```python
from build123d import *

# Parameters (mm, degrees)
F0_R           = 4.75
F0_R_2         = 8.6
F1_DEPTH       = 15.5
F2_R           = 7.25
F3_DEPTH       = 8
F4_R           = 23.5
F4_R_2         = 8.6
F5_DEPTH       = 27
F6_R           = 15.875
F7_DEPTH       = 8
F8_R           = 15.875
F9_DEPTH       = 10
F14_R          = 3
F15_DEPTH      = 25
F15_DEPTH_BACK = 25
F16_R          = 3
F17_DEPTH      = 15.5


with BuildPart() as f1:
    # F0 (on Front) → F1 (new body)
    with BuildSketch(Plane.XZ):
        with BuildLine():
            ThreePointArc((-54.5, -13.8241850861), (-27.977340312, -23.2893113667), (0, -26.5))
            ThreePointArc((0, -26.5), (27.977340312, -23.2893113667), (54.5, -13.8241850861))
            Line((54.5, -13.8241850861), (54.5, 12.5))
            Line((54.5, 12.5), (47.5, 12.5))
            Line((47.5, 12.5), (47.5, 17))
            ThreePointArc((47.5, 17), (0, 26.5), (-47.5, 17))
            Line((-47.5, 17), (-47.5, 12.5))
            Line((-47.5, 12.5), (-54.5, 12.5))
            Line((-54.5, 12.5), (-54.5, -13.8241850861))
        make_face()
        with Locations((-40, 0)):
            Circle(F0_R, mode=Mode.SUBTRACT)
        Circle(F0_R_2, mode=Mode.SUBTRACT)
        with Locations((40, 0)):
            Circle(F0_R, mode=Mode.SUBTRACT)
    extrude(amount=F1_DEPTH)

    # F2 (on face) → F3 (cut)
    with BuildSketch(Plane.XZ.offset(15.5)):
        with Locations((-40, 0)):
            Circle(F2_R)
        with Locations((40, 0)):
            Circle(F2_R)
    extrude(amount=-F3_DEPTH, mode=Mode.SUBTRACT)

    # F4 (on face) → F5 (join)
    with BuildSketch(Plane.XZ.offset(15.5)):
        Circle(F4_R)
        Circle(F4_R_2, mode=Mode.SUBTRACT)
    extrude(amount=F5_DEPTH)

    # F6 (on face) → F7 (cut)
    with BuildSketch(Plane.XZ.offset(42.5)):
        Circle(F6_R)
    extrude(amount=-F7_DEPTH, mode=Mode.SUBTRACT)

    # F8 (on face) → F9 (cut)
    with BuildSketch(Plane(origin=(0, 0, 0), x_dir=(-1, 0, 0), z_dir=(0, 1, 0))):
        Circle(F8_R)
    extrude(amount=-F9_DEPTH, mode=Mode.SUBTRACT)

    # F14 (on 3pt) → F15 (cut, two sides)
    with BuildSketch(Plane.XY.offset(-0.6620925431)) as f15_sk:
        with Locations((0, -21.5)):
            Circle(F14_R)
    extrude(amount=F15_DEPTH, mode=Mode.SUBTRACT)
    extrude(f15_sk.sketch, amount=-F15_DEPTH_BACK, mode=Mode.SUBTRACT)

    # F16 (on face) → F17 (cut, through all)
    with BuildSketch(Plane.XZ.offset(15.5)):
        with Locations((-31.9875436575, 13.577906715)):
            Circle(F16_R)
        with Locations((31.9875436575, -13.577906715)):
            Circle(F16_R)
    extrude(amount=-F17_DEPTH, mode=Mode.SUBTRACT)


solid = f1.part
```
For this review, take the finished solid that the model builds, in its own axes (mm). A direction names the side the tool comes from. Give positions to 0.01 mm unless a question says otherwise; leave off trailing zeros. Loops run counter-clockwise (first coordinate to the right, second up) from the corner with the lowest first, then second, coordinate; pieces in that order, holes last. Notation, with made-up numbers: M -31,-6 L 10,-6 A15 ccw 10,11 Z; hole C -17.5,43 d4. An arc over 180 degrees is marked long. One line per item, written item: value. Start each with the question number.
Q1. Add section C-C (y = -21.5). Give the boundary of the cut face in (x, z).
Q2. Add section D-D (x = -18.5). Give the boundary of the cut face in (y, z).
Q3. Add section A-A (x = 40). Give the boundary of the cut face in (y, z).
Q4. Draft analysis for pull direction Z (two halves, no side actions). For faces 4 (the face through (44.53, -3.7, 1.43)), 5 (the face through (-0.65, -24.43, 15.68)), 6 (the face through (-51, -8, 12.5)), state which applies: released by +Z, released by -Z, zero draft, split by the parting line, or undercut.
Q5. Clearance check with flat-ended pins moving along their axes: pin 1 Ø12 at (y, z) = (-20, 17.5) entering from -X; pin 2 Ø5 at (x, z) = (-10.5, 8) entering from -Y; pin 3 Ø22.5 at (x, z) = (0, 0) entering from +Y; pin 4 Ø9.5 at (x, z) = (-0.5, -3.5) entering from +Y. State where each tip first meets the part, or that it passes through.
Q6. Machinability: for faces 1 (the face through (51, -8, 12.5)), 2 (the face through (-7, -10, -7)), 3 (the face through (7, -34.5, -7)), which of the approach directions +Z, -Z, +X, -X, +Y, -Y give a long, thin tool a straight path to every point of the face, cutting with its end or side? Answer none if there is none.
Q7. Add section B-B (y = -2.5). Give the boundary of the cut face in (x, z) (3 decimals).
Q8. For L1, parallel to Y at x = 0, z = 20; L2, parallel to Y at x = 30.5, z = -10; L3, parallel to Z at x = 9, y = -7, list the stretches that pass through material, from the lowest coordinate up.
Reply:
1. outline: M -3,-23.31 L -3,-8.06 A8.6 cw -3,8.06 L -3,23.31 A23.5 ccw Z; M 3,-23.31 A23.5 ccw 3,23.31 L 3,8.06 A8.6 cw 3,-8.06 Z
2. outline: M -42.5,-14.49 L -15.5,-14.49 L -15.5,-25.11 L 0,-25.11 L 0,25.11 L -15.5,25.11 L -15.5,14.49 L -42.5,14.49 Z
3. outline: M -15.5,-19.84 L 0,-19.84 L 0,-4.75 L -7.5,-4.75 L -7.5,-7.25 L -15.5,-7.25 Z; M -15.5,7.25 L -7.5,7.25 L -7.5,4.75 L 0,4.75 L 0,19.84 L -15.5,19.84 Z
4. face 4: undercut
4. face 5: zero draft
4. face 6: released by +Z
5. pin 1: x = -47.5
5. pin 2: y = -34.5
5. pin 3: y = -10
5. pin 4: through
6. face 1: +Z, +X, +Y, -Y
6. face 2: +Y
6. face 3: -Y
7. outline: M -54.5,-13.824 A123.5 ccw 54.5,-13.824 L 54.5,12.5 L 47.5,12.5 L 47.5,17 A123.5 ccw -47.5,17 L -47.5,12.5 L -54.5,12.5 Z; hole C -40,0 d9.5; hole C -31.988,13.578 d6; hole C 0,0 d31.75; hole C 31.988,-13.578 d6; hole C 40,0 d9.5
8. L1: -42.5 to -24.5, -18.5 to 0
8. L2: -15.5 to 0
8. L3: -26.17 to -13.08, 13.08 to 26.17
